Input: part model. Units: mm. Frame: model coordinates. Face numbers are marked on the shaded views. A direction names the side the tool comes from. Round coordinates to 2 decimals unless told otherwise and drop trailing zeros. Loops run counter-clockwise (first coordinate to the right, second up) from the corner with the lowest first, then second, coordinate; pieces in that order, holes last. Notation, with made-up numbers: (40, -37) -> (85, -37) arc R23 ccw to (85, -23) -> close; hole circle Ø5 at (71, 55.25). An arc over 180 degrees is marked (long way). Answer in a Markdown table with one row per item. Add a question column.
Q1. Section B-B, the plane x = -30. Output: boundary loops of the cut face in (y, z), and give its area (3 significant figures).
Q2. Reachability of the marked faces 1, 2, 3, 4 and 5 from +Z, -Z, +X, -X, +Y, -Y: full face, straight path, thin tool, end or side. Return the list, or none.
Q3. Section A-A, the plane z = 0. Output: boundary loops of the cut face in (x, y).
Q4. Ray query, L1, parallel to Y at x = -6, z = 12.5; L2, parallel to Z at x = 34.5, y = 15; L3, parallel to Z at x = -41, y = -6. Return the intervals inside material, ascending. Write a range as from..to.
Q5. Mould query, pull axis Z, two halves, no side actions, for the marked faces 6, 7, 8 and 9. Classes: pulls with the +Z half, pulls with the -Z half, needs draft (parallel to the pull), parting line crosses it, or undercut.
Q6. Pin query (flat end, axial travel): pin 1 (1.6 mm diameter, centred on x = -39, y = -2, fed in from +Z); pin 2 (1 mm diameter, centred on x = 11, z = 5.5, fed in from -Y). Return the tip coordinate at first contact, or that it passes through.
Q7. Section C-C, the plane z = 14.5. Output: boundary loops of the cut face in (x, y).
```python
from build123d import *

# Parameters (mm, degrees)
SKETCH1_W           = 74.5
SKETCH1_H           = 40
BOSS_EXTRUDE1_DEPTH = 10
BOSS_EXTRUDE2_DEPTH = 6
BOSS_EXTRUDE3_DEPTH = 86.5


with BuildPart() as part:
    # Sketch1 → Boss-Extrude1 (new body)
    with BuildSketch(Plane(origin=(0, 0, 0), x_dir=(1, 0, 0), z_dir=(0, 1, 0))):
        Rectangle(SKETCH1_W, SKETCH1_H)
    extrude(amount=BOSS_EXTRUDE1_DEPTH)

    # Sketch2 → Boss-Extrude2 (add)
    # profile 1 of 2: a face of its own
    with BuildSketch(Plane(origin=(37.25, 0, 0), x_dir=(0, 0, -1), z_dir=(1, 0, 0))):
        with BuildLine():
            Line((7.5, 0), (-7.5, 0))
            Line((-7.5, 0), (-7.5, -5.45))
            ThreePointArc((-7.5, -5.45), (-7.280330086, -5.980330086), (-6.75, -6.2))
            Line((-6.75, -6.2), (-6.708203932, -6.2))
            ThreePointArc((-6.708203932, -6.2), (-6.208203932, -6.390983006), (-5.96284794, -6.866666667))
            ThreePointArc((-5.96284794, -6.866666667), (0, -12.2), (5.96284794, -6.866666667))
            ThreePointArc((5.96284794, -6.866666667), (6.208203932, -6.390983006), (6.708203932, -6.2))
            Line((6.708203932, -6.2), (6.75, -6.2))
            ThreePointArc((6.75, -6.2), (7.280330086, -5.980330086), (7.5, -5.45))
            Line((7.5, -5.45), (7.5, 0))
        make_face()
        with BuildLine():
            ThreePointArc((3, -6.2), (0, -9.2), (-3, -6.2))
            ThreePointArc((-3, -6.2), (0, -3.2), (3, -6.2))
        make_face(mode=Mode.SUBTRACT)
    # profile 2 of 2: a face of its own
    with BuildSketch(Plane(origin=(37.25, 0, 0), x_dir=(0, 0, -1), z_dir=(1, 0, 0))):
        Polygon((-20, 0), (-7.5, 0), (7.5, 0), (20, 0), (20, 10), (-20, 10), align=None)
    boss_extrude2 = extrude(amount=BOSS_EXTRUDE2_DEPTH)

    # Mirror1: Boss-Extrude2 across plane
    add(boss_extrude2.mirror(Plane(origin=(0, 0, 0), x_dir=(0, 0, 1), z_dir=(1, 0, 0))))

    # Sketch3 → Boss-Extrude3 (add)
    with BuildSketch(Plane.ZY.offset(43.25)):
        with BuildLine():
            Line((-3.838227356, 14.8), (-3.838227356, 10))
            Line((-3.838227356, 10), (3.838227356, 10))
            Line((3.838227356, 10), (3.838227356, 14.8))
            Line((3.838227356, 14.8), (7.238227356, 14.8))
            Line((7.238227356, 14.8), (7.238227356, 14.3))
            ThreePointArc((7.238227356, 14.3), (7.531120575, 13.592893219), (8.238227356, 13.3))
            Line((8.238227356, 13.3), (9.438227356, 13.3))
            Line((9.438227356, 13.3), (9.438227356, 14.8))
            Line((9.438227356, 14.8), (9.438227356, 18.08))
            Line((9.438227356, 18.08), (5.3521045, 21.88))
            Line((5.3521045, 21.88), (-5.3521045, 21.88))
            Line((-5.3521045, 21.88), (-9.438227356, 18.08))
            Line((-9.438227356, 18.08), (-9.438227356, 14.8))
            Line((-9.438227356, 14.8), (-9.438227356, 13.3))
            Line((-9.438227356, 13.3), (-8.238227356, 13.3))
            ThreePointArc((-8.238227356, 13.3), (-7.531120575, 13.592893219), (-7.238227356, 14.3))
            Line((-7.238227356, 14.3), (-7.238227356, 14.8))
            Line((-7.238227356, 14.8), (-3.838227356, 14.8))
        make_face()
    extrude(amount=-BOSS_EXTRUDE3_DEPTH)


solid = part.part
```
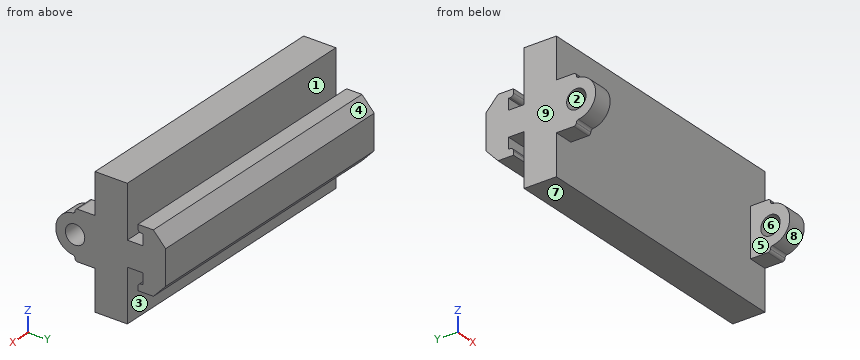
Answer block:
| question | item | result |
|---|---|---|
| 1 | outline | (0, -20) -> (10, -20) -> (10, -3.84) -> (14.8, -3.84) -> (14.8, -7.24) -> (14.3, -7.24) arc R1 ccw to (13.3, -8.24) -> (13.3, -9.44) -> (18.08, -9.44) -> (21.88, -5.35) -> (21.88, 5.35) -> (18.08, 9.44) -> (13.3, 9.44) -> (13.3, 8.24) arc R1 ccw to (14.3, 7.24) -> (14.8, 7.24) -> (14.8, 3.84) -> (10, 3.84) -> (10, 20) -> (0, 20) -> close |
| 1 | area | 561 mm^2 |
| 2 | face 1 | +Z, +X, -X |
| 2 | face 2 | +X, -X |
| 2 | face 3 | -Z, +X, -X |
| 2 | face 4 | +Z, +X, -X, +Y |
| 2 | face 5 | +Z, -Z, -Y |
| 3 | outline | (-43.25, -12.2) -> (-37.25, -12.2) -> (-37.25, -9.2) -> (-43.25, -9.2) -> close; (-43.25, -3.2) -> (-37.25, -3.2) -> (-37.25, 0) -> (37.25, 0) -> (37.25, -3.2) -> (43.25, -3.2) -> (43.25, 21.88) -> (-43.25, 21.88) -> close; (37.25, -12.2) -> (43.25, -12.2) -> (43.25, -9.2) -> (37.25, -9.2) -> close |
| 4 | L1 | 0..10 |
| 4 | L2 | -9.44..9.44 |
| 4 | L3 | -7.26..-2.99, 2.99..7.26 |
| 5 | face 6 | undercut |
| 5 | face 7 | pulls with the -Z half |
| 5 | face 8 | parting line crosses it |
| 5 | face 9 | needs draft |
| 6 | pin 1 | z = 7.5 |
| 6 | pin 2 | y = 0 |
| 7 | outline | (-43.25, 0) -> (43.25, 0) -> (43.25, 10) -> (-43.25, 10) -> close |
